Can you work these out from the model? Positions are in its coordinate system, mm. A direction names the side the tool comes from. Round coordinates to 2 decimals unless told otherwise and drop trailing zeros. Order: outer loops, then holes, each group sorted by start corner. A loop starts at its lowest first (then second) coordinate and runs counter-clockwise, first axis right, second up. Notation, with made-up numbers: (25, 31.25) -> (39, 31.25) arc R25 cw to (39, 49.25) -> close; hole circle Ø5 at (-12, 80). An arc over 180 degrees is marked (long way). One line per item, written item: value.
```python
from build123d import *

# Parameters (mm, degrees)
BOSS_EXTRUDE1_DEPTH = 7
BOSS_EXTRUDE2_DEPTH = 28


with BuildPart() as part:
    # Sketch1 → Boss-Extrude1 (new body)
    with BuildSketch(Plane(origin=(0, 0, 0), x_dir=(1, 0, 0), z_dir=(0, 1, 0))):
        with BuildLine():
            Line((50, 28), (28, 28))
            Line((28, 28), (28, 0))
            Line((28, 0), (50, 0))
            Line((50, 0), (50, 7))
            Line((50, 7), (43, 7))
            ThreePointArc((43, 7), (36, 14), (43, 21))
            Line((43, 21), (50, 21))
            Line((50, 21), (50, 28))
        make_face()
    extrude(amount=BOSS_EXTRUDE1_DEPTH)

    # Sketch1<3> → Boss-Extrude2 (add)
    with BuildSketch(Plane(origin=(0, 0, 0), x_dir=(1, 0, 0), z_dir=(0, 1, 0))):
        Polygon((0, 28), (0, 0), (7, 0), (7, 21), (21, 21), (21, 0), (28, 0), (28, 28), align=None)
    extrude(amount=BOSS_EXTRUDE2_DEPTH)


solid = part.part
```
Q1. On a 3-axis mill with a long thin cutter (end or side, diameter ignored), from which of +Z, -Z, +X, -X, +Y, -Y can I reach the whole of each face in a straight line? I mean faces 4 (the face through (21, 14, -11)), 5 (the face through (47, 3, -7)), 6 (the face through (0, 14, -14)), 7 (the face through (34, 7, -14)). Say none if no direction works.
Answers below:
face 4: +Z, +Y, -Y
face 5: +X, +Y, -Y
face 6: +Z, -Z, -X, +Y, -Y
face 7: +Z, -Z, +X, +Y
Q2. We'd pull the mould along Z, two halves only. Please class faces 1 (the face through (14, 14, -21)), 2 (the face through (7, 14, -10)), 3 (the face through (46, 3, -21)): released by +Z, released by -Z, zero draft, split by the parting line, or undercut.
Answers below:
face 1: released by +Z
face 2: zero draft
face 3: undercut
Q3. I want a section at B-B on y = 2. List the corners of the cut face in (x, z) for me.
Answers below:
outline: (0, -28) -> (50, -28) -> (50, -21) -> (43, -21) arc R7 cw to (43, -7) -> (50, -7) -> (50, 0) -> (21, 0) -> (21, -21) -> (7, -21) -> (7, 0) -> (0, 0) -> close
Q4. I want a section at A-A on z = -14. List the corners of the cut face in (x, y) for me.
Answers below:
outline: (0, 0) -> (7, 0) -> (7, 28) -> (0, 28) -> close; (21, 0) -> (36, 0) -> (36, 7) -> (28, 7) -> (28, 28) -> (21, 28) -> close
Q5. Please list where these lines run through material, in increasing order: line 1 along X through (y, z) = (3.5, -2.5); line 2 along X through (y, z) = (7.5, -5); line 3 along Z through (x, y) = (46, 6.5).
Answers below:
line 1: 0 to 7, 21 to 50
line 2: 0 to 7, 21 to 28
line 3: -28 to -21, -7 to 0
Q6. Will these pins go through, and if not, where does the flat tip stop? pin 1 Ø10 at (x, z) = (13, -4) entering from -Y; pin 2 Ø1 at (x, z) = (34.5, -20.5) entering from +Y; pin 3 Ø10.5 at (y, z) = (15, -9) entering from +X.
Answers below:
pin 1: through
pin 2: y = 7
pin 3: x = 28
Q7. I want a section at C-C on z = -24.75. List the corners of the cut face in (x, y) for me.
Answers below:
outline: (0, 0) -> (50, 0) -> (50, 7) -> (28, 7) -> (28, 28) -> (0, 28) -> close
Q8. I want a section at D-D on z = -1.75. List the corners of the cut face in (x, y) for me.
Answers below:
outline: (0, 0) -> (7, 0) -> (7, 28) -> (0, 28) -> close; (21, 0) -> (50, 0) -> (50, 7) -> (28, 7) -> (28, 28) -> (21, 28) -> close
